Work out the finished part from the listing and answer in its coordinate system (mm). A direction names the side the tool comes from. Give positions to 0.01 mm unless a question says otherwise; leave off trailing zeros. Order: outer loops, then holes, each group sorted by start corner. A loop starts at its lowest first (then second) coordinate and runs counter-clockwise, first axis right, second up. Notation, with made-up numbers: (48, 83.25) -> (70, 83.25) arc R15 ccw to (70, 111.25) -> close; hole circle Ø10 at (11.25, 35). An arc over 180 degrees is marked (long way). Answer as CSV lines item,"result". Start each with the question number.
1. For a pull along Y with two mould halves and no side action, classify faces 6 (the flat face through (0, 0, -5)), 7 (the cylindrical face through (-27.01, 27.28, -0.27)), 8 (the cylindrical face through (0.27, 0.99, -5.78)), 9 (the cylindrical face through (26.99, 17.78, -0.27)) as released by +Y, released by -Y, zero draft, split by the parting line, or undercut.
2. A cutting plane is placed at A-A (y = 9.5). Give the vertices of the cut face in (x, z) (3 decimals), then the cut area to 3 significant figures.
3. For faces 1 (the flat face through (22, 6, -3.175)), 2 (the flat face through (0, 2, -5)), 3 (the flat face through (-15, 2, 0)), 4 (the cylindrical face through (-27.01, 51.24, -7.16)), 5 (the flat face through (-19.2, 8.9, 0)), determine the directions among +Z, -Z, +X, -X, +Y, -Y from which every point of the face is accessible in a straight line to the end or side of a thin tool.
4. A cutting plane is placed at C-C (x = -7). Give the vertices of the cut face in (y, z).
5. Find the intervals of material crossed by L1, parallel to X at y = 14, z = 9.25; L2, parallel to Z at x = 7, y = 1; L3, parallel to X at y = 0.7, z = 7, in increasing order.
6. A cutting plane is placed at D-D (x = -24). Give the vertices of the cut face in (y, z) (3 decimals).
7. A cutting plane is placed at B-B (y = 43). Give the vertices of the cut face in (x, z).
8. Flat-ended cylindrical pins translate along their axes: pin 1 (7 mm diameter, centred on x = -20, y = 7.5, fed in from -Z) (3 decimals); pin 2 (10 mm diameter, centred on x = -11.5, z = -1.5, fed in from +Y); pin 3 (5 mm diameter, centred on x = -10, z = 7.5, fed in from +Y). Find the tip coordinate at first contact, or state that the pin passes through.
from build123d import *

# Parameters (mm, degrees)
T_LE_DE_BASE_PLI_E1_DEPTH       = 12
ENL_V_START                     = -56
ENL_V_MAT_EXTRU_1_DEPTH         = 56
DIAM_TRE_DU_PER_AGE_8_0_8_1_D   = 8
DIAM_TRE_DU_PER_AGE_2_5_2_5_1_D = 2.5
DIAM_TRE_DU_PER_AGE_8_0_8_2_D   = 8
DIAM_TRE_DU_PER_AGE_2_5_2_5_2_D = 2.5
BOSS_EXTRUDE1_DEPTH             = 3.175


# Read off the part's stored shape, not the designer's step: Enlèv. mat.-Extru.1
# Sheet-metal steps are written as plain solids
with BuildPart() as part:
    # Esquisse1 → Tôle de base pliée1 (new, symmetric)
    with BuildSketch(Plane.XY):
        with BuildLine():
            Line((-28, 62), (-28, 3))
            ThreePointArc((-28, 3), (-27.121320344, 0.878679656), (-25, 0))
            Line((-25, 0), (25, 0))
            ThreePointArc((25, 0), (27.121320344, 0.878679656), (28, 3))
            Line((28, 3), (28, 62))
            Line((28, 62), (26, 62))
            Line((26, 62), (26, 3))
            ThreePointArc((26, 3), (25.707106781, 2.292893219), (25, 2))
            Line((25, 2), (-25, 2))
            ThreePointArc((-25, 2), (-25.707106781, 2.292893219), (-26, 3))
            Line((-26, 3), (-26, 62))
            Line((-26, 62), (-28, 62))
        make_face()
    extrude(amount=T_LE_DE_BASE_PLI_E1_DEPTH, both=True)

    # Enlèv. mat.-Extru.1 outline → Enlèv. mat.-Extru.1 (cut)
    with BuildSketch(Plane(origin=(28, 0, 0), x_dir=(0, 0, -1), z_dir=(1, 0, 0)).offset(ENL_V_START)):
        with BuildLine():
            ThreePointArc((-12, 50), (-8.485281374, 58.485281374), (0, 62))
            Line((0, 62), (-12, 62))
            Line((-12, 62), (-12, 50))
        make_face()
        with BuildLine():
            ThreePointArc((0, 62), (8.485281374, 58.485281374), (12, 50))
            Line((12, 50), (12, 62))
            Line((12, 62), (0, 62))
        make_face()
    extrude(amount=ENL_V_MAT_EXTRU_1_DEPTH, mode=Mode.SUBTRACT)

    # Diamètre du perçage Ø8.0 (8)1 (through all)
    with Locations(Plane(origin=(28, 0, 0), x_dir=(0, 0, -1), z_dir=(1, 0, 0))):
        with Locations((0, 50)):
            Hole(DIAM_TRE_DU_PER_AGE_8_0_8_1_D / 2)

    # Diamètre du perçage Ø2.5 (2.5)1 (through all)
    with Locations(Plane(origin=(28, 0, 0), x_dir=(0, 0, -1), z_dir=(1, 0, 0))):
        with Locations((0, 57), (7, 50), (0, 43), (-7, 50), (0, 34.5), (0, 28.5), (0, 19)):
            Hole(DIAM_TRE_DU_PER_AGE_2_5_2_5_1_D / 2)

    # Diamètre du perçage Ø8.0 (8)2 (through all)
    with Locations(Plane(origin=(0, 2, 0), x_dir=(1, 0, 0), z_dir=(0, 1, 0))):
        with Locations((0, 0)):
            Hole(DIAM_TRE_DU_PER_AGE_8_0_8_2_D / 2)

    # Diamètre du perçage Ø2.5 (2.5)2 (through all)
    with Locations(Plane(origin=(0, 2, 0), x_dir=(1, 0, 0), z_dir=(0, 1, 0))):
        with Locations((0, 7), (7, 0), (0, -7), (-7, 0), (-15.5, 0), (15.5, 0)):
            Hole(DIAM_TRE_DU_PER_AGE_2_5_2_5_2_D / 2)

    # Sketch1 → Boss-Extrude1 (add, symmetric)
    with BuildSketch(Plane(origin=(0, 0, 0), x_dir=(-1, 0, 0), z_dir=(0, 0, -1))):
        with BuildLine():
            Line((26, 15.7), (12.3, 2))
            Line((12.3, 2), (25, 2))
            ThreePointArc((25, 2), (25.707106781, 2.292893219), (26, 3))
            Line((26, 3), (26, 15.7))
        make_face()
    boss_extrude1 = extrude(amount=BOSS_EXTRUDE1_DEPTH, both=True)

    # Mirror1: Boss-Extrude1 across plane
    add(boss_extrude1.mirror(Plane(origin=(0, 0, 0), x_dir=(0, 0, 1), z_dir=(1, 0, 0))))


solid = part.part
Answer sheet:
1,face 6,"released by -Y"
1,face 7,"undercut"
1,face 8,"zero draft"
1,face 9,"undercut"
2,outline,"(-28, -12) -> (-26, -12) -> (-26, -3.175) -> (-19.8, -3.175) -> (-19.8, 3.175) -> (-26, 3.175) -> (-26, 12) -> (-28, 12) -> close; (19.8, -3.175) -> (26, -3.175) -> (26, -12) -> (28, -12) -> (28, 12) -> (26, 12) -> (26, 3.175) -> (19.8, 3.175) -> close"
2,area,"175 mm^2"
3,face 1,"-Z, +Y"
3,face 2,"+Y"
3,face 3,"-Y"
3,face 4,"+X, -X"
3,face 5,"+Z, -Z, +Y"
4,outline,"(0, -12) -> (2, -12) -> (2, -1.25) -> (0, -1.25) -> close; (0, 1.25) -> (2, 1.25) -> (2, 12) -> (0, 12) -> close"
5,L1,"x = -28 to -26, 26 to 28"
5,L2,"z = -12 to -1.25, 1.25 to 12"
5,L3,"x = -26.93 to -1.25, 1.25 to 26.93"
6,outline,"(0, -12) -> (2, -12) -> (2, -3.175) -> (13.7, -3.175) -> (13.7, 3.175) -> (2, 3.175) -> (2, 12) -> (0, 12) -> close"
7,outline,"(-28, -12) -> (-26, -12) -> (-26, -1.25) -> (-28, -1.25) -> close; (-28, 1.25) -> (-26, 1.25) -> (-26, 12) -> (-28, 12) -> close; (26, -12) -> (28, -12) -> (28, -1.25) -> (26, -1.25) -> close; (26, 1.25) -> (28, 1.25) -> (28, 12) -> (26, 12) -> close"
8,pin 1,"stops at z = -3.175"
8,pin 2,"stops at y = 6.2"
8,pin 3,"stops at y = 2"
